Input: dimensioned drawing with shaded views. Units: mm. Origin: part minimum x, y, z. Round coordinates to 2 decimals unless told otherwise and drop trailing zeros. Loops run counter-clockwise (first coordinate to the right, second up) from the corner with the lowest first, then second, coordinate; pieces in that order, holes last. Notation, with made-up numbers: (-2, 63.25) - (2, 63.25) arc R16 cw to (2, 91.25) - close; hole circle Ø8 at (20, 81.5). An arc over 180 degrees is marked (long way). One line per question, with ' | ' between items.
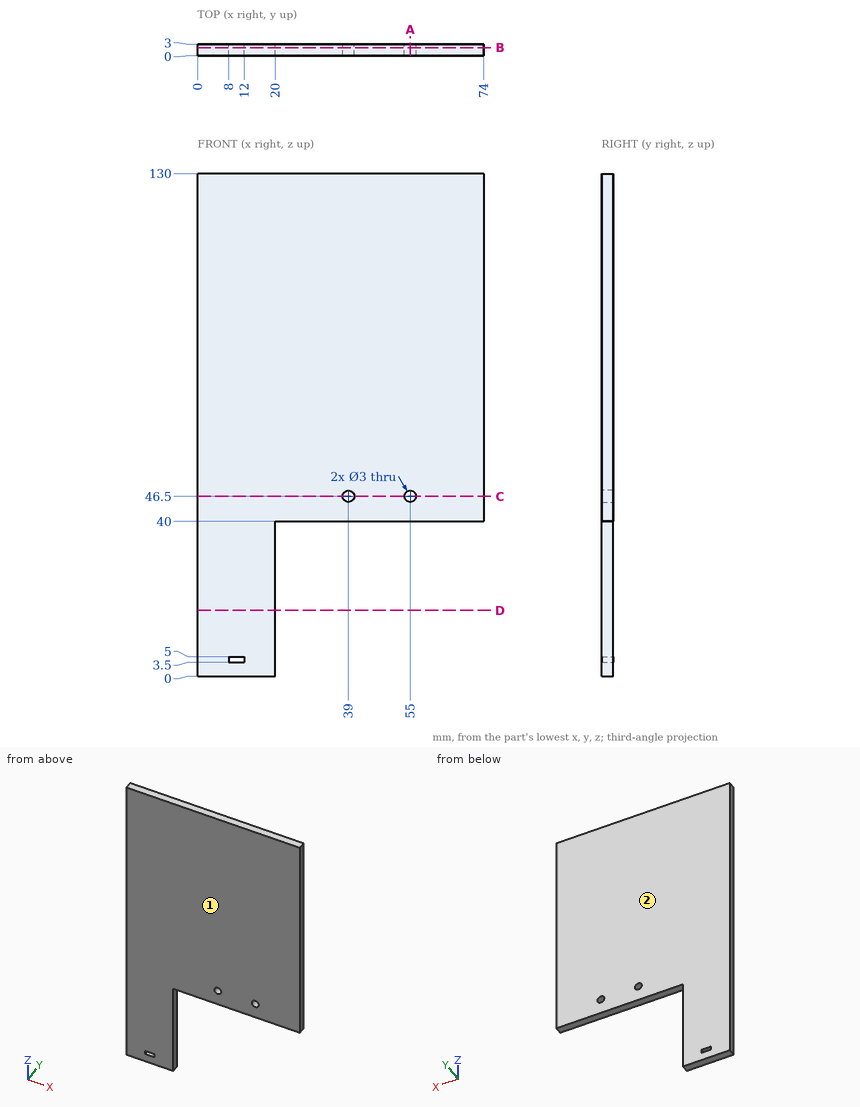
1. Contact query for flat-ended pins moving along their axis: P1, Ø8, axis at x = 37, z = 103.5, coming from the -Y side; P2, Ø1.5, axis at x = 62.5, y = 1.5, coming from the -Z side; P3, Ø2.5, axis at x = 39, z = 46.5, coming from the -Y side; P4, Ø0.9, axis at y = 1, z = 15.5, coming from the +X side. Output: stop coordinate, or through.
Worked out:
P1: stops at y = 0 | P2: stops at z = 40 | P3: passes through | P4: stops at x = 20
2. Section query A-A, the plane x = 55. Return loops of the section in (y, z).
Worked out:
outline: (0, 40) - (3, 40) - (3, 45) - (0, 45) - close; (0, 48) - (3, 48) - (3, 130) - (0, 130) - close
3. Section query C-C, the plane z = 46.5. Return loops of the section in (x, y).
Worked out:
outline: (0, 0) - (37.5, 0) - (37.5, 3) - (0, 3) - close; (40.5, 0) - (53.5, 0) - (53.5, 3) - (40.5, 3) - close; (56.5, 0) - (74, 0) - (74, 3) - (56.5, 3) - close
4. Mould query, pull axis Y, two halves, no side actions, for the marked faces 1 and 2. Classes: released by +Y, released by -Y, zero draft, split by the parting line, or undercut.
Worked out:
face 1: released by -Y | face 2: released by +Y
5. Material intervals for probe 1 along X at (y, z) = (1.8, 46.5); probe 2 along X at (y, z) = (1.1, 24.5); probe 3 along Z at (x, y) = (25, 2.5), sorted ascending.
Worked out:
probe 1: x = 0 to 37.5, 40.5 to 53.5, 56.5 to 74 | probe 2: x = 0 to 20 | probe 3: z = 40 to 130
6. Section query B-B, the plane y = 2.05. Return loops of the section in (x, z).
Worked out:
outline: (0, 0) - (20, 0) - (20, 40) - (74, 40) - (74, 130) - (0, 130) - close; hole (8, 3.5) - (12, 3.5) - (12, 5) - (8, 5) - close; hole circle Ø3 at (39, 46.5); hole circle Ø3 at (55, 46.5)
7. Section query D-D, the plane z = 17. Return loops of the section in (x, y).
Worked out:
outline: (0, 0) - (20, 0) - (20, 3) - (0, 3) - close
